from build123d import *

# Parameters (mm, degrees)
SKETCH2_R           = 50
BOSS_EXTRUDE1_DEPTH = 3
SKETCH3_R           = 5
BOSS_EXTRUDE2_DEPTH = 10
FILLET1_R           = 5


with BuildPart() as part:
    # Sketch2 → Boss-Extrude1 (new body)
    with BuildSketch(Plane(origin=(0, 0, 0), x_dir=(1, 0, 0), z_dir=(0, 1, 0))):
        with Locations(Location((0, 0, 0), (0, 0, 270))):
            Circle(SKETCH2_R)
    extrude(amount=BOSS_EXTRUDE1_DEPTH)

    # Sketch3 → Boss-Extrude2 (add)
    with BuildSketch(Plane(origin=(0, 3, 0), x_dir=(1, 0, 0), z_dir=(0, 1, 0))):
        with Locations(Location((0, 0, 0), (0, 0, 270))):
            Circle(SKETCH3_R)
        with BuildLine():
            Line((2, 1.5), (2, -1.5))
            ThreePointArc((2, -1.5), (-2.5, 0), (2, 1.5))
        make_face(mode=Mode.SUBTRACT)
    extrude(amount=BOSS_EXTRUDE2_DEPTH)

    # Fillet1
    fillet1_edges = [part.edges().sort_by_distance(p)[0] for p in [
        (0, 3, -5),
    ]]
    fillet(fillet1_edges, radius=FILLET1_R)


solid = part.part
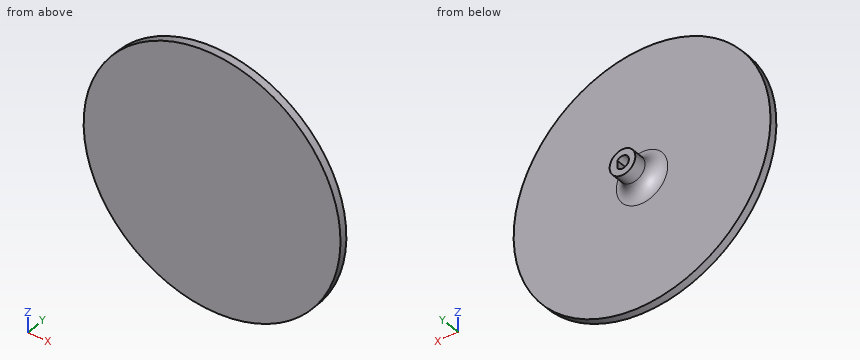
Geometry check sheet. Reference: the model listing, model coordinates, mm. Round coordinates to 2 decimals unless told otherwise and drop trailing zeros. Write each loop counter-clockwise with the first axis right and the second up, starting at its lowest first coordinate (ties: lowest second). Pieces come first, ordered by that corner, then holes.
Item 1: Material ranges on line 1 along Y through (x, z) = (-24, 3.5); line 2 along Z through (x, y) = (38.5, 1.25); line 3 along X through (y, z) = (2.5, -24), recorded low to high.
Determined:
line 1: y = 0 to 3
line 2: z = -31.9 to 31.9
line 3: x = -43.86 to 43.86
Item 2: Go/stop test with flat-tipped pins: pin 1 Ø3 at (x, y) = (-6, 1.5) entering from -Z; pin 2 Ø2 at (x, z) = (6, -34) entering from +Y; pin 3 Ø4 at (y, z) = (4.5, -16.5) entering from +X. Record where each tip stops, or that it passes through.
Determined:
pin 1: stops at z = -49.8
pin 2: stops at y = 3
pin 3: stops at x = 47.64
Item 3: Section check B-B (z = 0). Record the boundary of the cut face in (x, y), plus the area to 3 significant figures.
Determined:
outline: (-50, 0) - (50, 0) - (50, 3) - (10, 3) arc R5 cw to (5, 8) - (5, 13) - (2, 13) - (2, 3) - (-2.5, 3) - (-2.5, 13) - (-5, 13) - (-5, 8) arc R5 cw to (-10, 3) - (-50, 3) - close
area: 366 mm2
Item 4: Section check C-C (y = 11). Record the boundary of the cut face in (x, z), plus the area to 3 significant figures.
Determined:
outline: circle Ø10 at (0, 0); hole (2, -1.5) - (2, 1.5) arc R2.5 ccw (long way) to start
area: 59.9 mm2
Item 5: Section check A-A (x = 0). Record the boundary of the cut face in (y, z), plus the area to 3 significant figures.
Determined:
outline: (0, -50) - (3, -50) - (3, -10) arc R5 cw to (8, -5) - (13, -5) - (13, -2.5) - (3, -2.5) - (3, 2.5) - (13, 2.5) - (13, 5) - (8, 5) arc R5 cw to (3, 10) - (3, 50) - (0, 50) - close
area: 361 mm2
Item 6: Section check D-D (x = -30). Record the boundary of the cut face in (y, z), plus the area to 3 significant figures.
Determined:
outline: (0, -40) - (3, -40) - (3, 40) - (0, 40) - close
area: 240 mm2
